Build history of the part. All positions in model axes, mm. Face numbers are marked on the shaded views. A direction names the side the tool comes from. Coordinates: 2 decimals unless noted, no trailing zeros. Write each loop counter-clockwise with the first axis right and the second up, starting at its lowest first coordinate (ties: lowest second). Pieces come first, ordered by that corner, then holes.
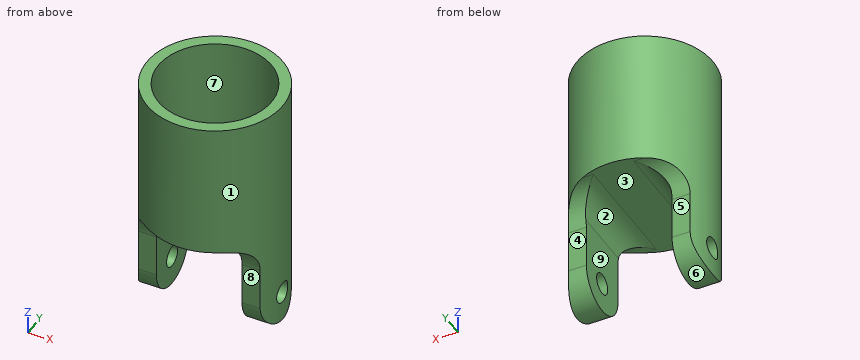
from build123d import *

# Parameters (mm, degrees)
CUT_EXTRUDE1_DEPTH      = 38.432697939
CUT_EXTRUDE1_DEPTH_BACK = 38.432697939
CUT_EXTRUDE2_DEPTH      = 38.432698083
CUT_EXTRUDE2_DEPTH_BACK = 38.432698083
SKETCH5_W               = 23.799010272
SKETCH5_H               = 22.882778694
CUT_EXTRUDE3_DEPTH      = 5.43
CUT_EXTRUDE4_DEPTH      = 25.43
CUT_EXTRUDE4_DEPTH_BACK = 15.43
SKETCH6_R               = 1.49


with BuildPart() as part:
    # Sketch1 → Revolve1 (revolve)
    with BuildSketch(Plane(origin=(0, 0, 0), x_dir=(0, 0, -1), z_dir=(1, 0, 0))):
        Polygon((-34.925, 9.525), (-34.925, 7.9375), (-15.925, 7.9375), (-15.925, 0), (9.525, 0), (9.525, 9.525), align=None)
    revolve(axis=Axis((0, 0, 0), (0, 0, 1)))

    # Sketch3 → Cut-Extrude1 (cut, two sides: drawn at the far end of the back side and taken through both)
    with BuildSketch(Plane(origin=(0, 0, 0), x_dir=(0, 0, -1), z_dir=(1, 0, 0)).offset(-CUT_EXTRUDE1_DEPTH_BACK)):
        with BuildLine():
            Line((9.525, 9.525), (-10.233333333, 9.525))
            Line((-10.233333333, 9.525), (-10.233333333, 8.466666667))
            ThreePointArc((-10.233333333, 8.466666667), (-8.993418707, 5.47324796), (-6, 4.233333333))
            Line((-6, 4.233333333), (0, 4.233333333))
            ThreePointArc((0, 4.233333333), (4.233333333, 0), (0, -4.233333333))
            Line((0, -4.233333333), (-6, -4.233333333))
            ThreePointArc((-6, -4.233333333), (-8.993418707, -5.47324796), (-10.233333333, -8.466666667))
            Line((-10.233333333, -8.466666667), (-10.233333333, -9.525))
            Line((-10.233333333, -9.525), (9.525, -9.525))
            Line((9.525, -9.525), (9.525, 9.525))
        make_face()
    extrude(amount=CUT_EXTRUDE1_DEPTH + CUT_EXTRUDE1_DEPTH_BACK, mode=Mode.SUBTRACT)

    # Sketch4 → Cut-Extrude2 (cut, two sides: drawn at the far end of the back side and taken through both)
    with BuildSketch(Plane(origin=(0, 0, 0), x_dir=(1, 0, 0), z_dir=(0, 1, 0)).offset(-CUT_EXTRUDE2_DEPTH_BACK)):
        with BuildLine():
            Line((-2.825, -10.233333333), (2.825, -10.233333333))
            ThreePointArc((2.825, -10.233333333), (5.07006403, -9.303397364), (6, -7.058333333))
            Line((6, -7.058333333), (6, 4.233333333))
            Line((6, 4.233333333), (-6, 4.233333333))
            Line((-6, 4.233333333), (-6, -7.058333333))
            ThreePointArc((-6, -7.058333333), (-5.07006403, -9.303397364), (-2.825, -10.233333333))
        make_face()
    extrude(amount=CUT_EXTRUDE2_DEPTH + CUT_EXTRUDE2_DEPTH_BACK, mode=Mode.SUBTRACT)

    # Sketch5 → Cut-Extrude3 (cut)
    with BuildSketch(Plane.XY.offset(34.925)):
        Rectangle(SKETCH5_W, SKETCH5_H)
    extrude(amount=-CUT_EXTRUDE3_DEPTH, mode=Mode.SUBTRACT)

    # Sketch6 → Cut-Extrude4 (cut, two sides: drawn at the far end of the back side and taken through both)
    with BuildSketch(Plane(origin=(-6, 0, 0), x_dir=(0, 0, -1), z_dir=(1, 0, 0)).offset(-CUT_EXTRUDE4_DEPTH_BACK)):
        with Locations(Location((0, 0, 0), (0, 0, 180))):
            Circle(SKETCH6_R)
    extrude(amount=CUT_EXTRUDE4_DEPTH + CUT_EXTRUDE4_DEPTH_BACK, mode=Mode.SUBTRACT)


solid = part.part
(1) Slice it at C-C, the plane x = 0. List the corners of the cut face in (y, z) (1 decimal), and give its area (3 significant figures).
(2) Probe L1, parallel to X at y = 0, z = 24 (1 decimal); L2, parallel to Y at x = -8, z = 0; L3, parallel to Z at x = -0.25, y = -6.5 (3 decimals). List the from-to ranges inside material, lowest first.
(3) Slice it at B-B, the plane z = 3.5. List the corners of the cut face in (x, y) (3 decimals).
(4) Two-plate mould, pull along X, no slides. Class the marked faces 1, 2, 3 and 4: pulls with the +X half, pulls with the -X half, needs draft (parallel to the pull), parting line crosses it, or undercut.
(5) 3-axis set-ups, long thin cutter, end or side, ignore diameter. For the marked faces 5, 6, 7, 8 and 9: which of +Z, -Z, +X, -X, +Y, -Y reach the whole face in a straight line?
(6) Slice it at A-A, the plane y = 0. Give the number of separate pieces and of enclosed holes in the cut face, and give its area (3 significant figures).
(7) Flat gauge pins, fed straight in: P1, Ø2, axis at x = -4, y = 4, coming from the +Z side (3 decimals); P2, Ø9.5, axis at y = 2, z = 4, coming from the -X side (3 decimals); P3, Ø3, axis at x = 6, z = 11, coming from the -Y side (3 decimals); P4, Ø0.8, axis at x = 7.5, z = 3, coming from the +Y side. Where does each tip first touch, or does it go through?
Results:
1. outline: (-9.5, 10.2) - (9.5, 10.2) - (9.5, 29.5) - (7.9, 29.5) - (7.9, 15.9) - (-7.9, 15.9) - (-7.9, 29.5) - (-9.5, 29.5) - close
1. area: 152 mm2
2. L1: x = -9.5 to -7.9, 7.9 to 9.5
2. L2: y = -4.23 to -1.49, 1.49 to 4.23
2. L3: z = 10.233 to 15.925
3. outline: (-8.533, -4.233) - (-6, -4.233) - (-6, 4.233) - (-8.533, 4.233) arc R9.525 ccw to start; (6, -4.233) - (8.533, -4.233) arc R9.525 ccw to (8.533, 4.233) - (6, 4.233) - close
4. face 1: parting line crosses it
4. face 2: undercut
4. face 3: undercut
4. face 4: needs draft
5. face 5: -Z, +X, -X, +Y
5. face 6: -Z, +X, -X
5. face 7: +Z
5. face 8: -Z, +X, -X, -Y
5. face 9: -Z, +Y, -Y
6. separate pieces: 3
6. enclosed holes: 0
6. area: 237 mm2
7. P1: stops at z = 15.925
7. P2: stops at x = -9.525
7. P3: stops at y = -8.395
7. P4: stops at y = 4.23
